The model under review builds one solid part; all positions refer to its coordinate system, in mm. Face numbers are marked on the shaded views. A direction names the side the tool comes from. Give positions to 0.01 mm unless a question says otherwise; leave off trailing zeros. Order: outer loops, then holes, each group sorted by start corner. A loop starts at its lowest first (then second) coordinate and runs counter-clockwise, first axis right, second up. Notation, with made-up numbers: (-38, -19.5) - (-33, -19.5) arc R19 ccw to (-33, -0.5) - close; hole circle Ø4 at (60.5, 80). An arc over 180 degrees is marked (long way). Use a Markdown table: item, result. Add a question column.
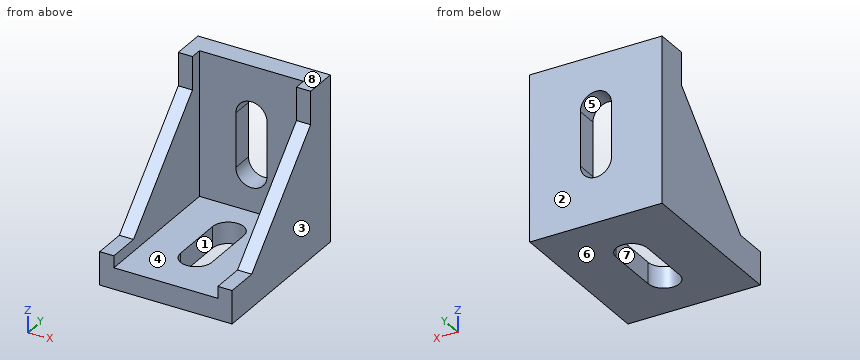
```python
from build123d import *

# Parameters (mm, degrees)
PAD_DEPTH            = 14
BOX_W                = 33
BOX_H                = 33
BOX_DEPTH            = 22
POCKET_DEPTH         = 4.5
POCKET001_DEPTH      = 4.5
BODY_ROLL_ANGLE      = 90
BODY_PLACEMENT_ANGLE = -90


with BuildPart() as part:
    # Sketch → Pad (new body, symmetric)
    with BuildSketch(Plane.XY):
        Polygon((0, 0), (0, 35), (7, 35), (7, 28), (28, 7), (35, 7), (35, 0), align=None)
    extrude(amount=PAD_DEPTH, both=True)

    # Box → Box (cut)
    with BuildSketch(Plane(origin=(4.5, 4.5, -11), x_dir=(1, 0, 0), z_dir=(0, 0, 1))):
        with Locations((16.5, 16.5)):
            Rectangle(BOX_W, BOX_H)
    extrude(amount=BOX_DEPTH, mode=Mode.SUBTRACT)

    # Sketch001 (on Face1 of Box) → Pocket (cut)
    with BuildSketch(Plane(origin=(0, 0, 0), x_dir=(0, -1, 0), z_dir=(-1, 0, 0))):
        with BuildLine():
            ThreePointArc((-24.2, 3.3), (-27.5, 0), (-24.2, -3.3))
            Line((-24.2, -3.3), (-12.8, -3.3))
            ThreePointArc((-12.8, -3.3), (-9.5, 0), (-12.8, 3.3))
            Line((-24.2, 3.3), (-12.8, 3.3))
        make_face()
    extrude(amount=-POCKET_DEPTH, mode=Mode.SUBTRACT)

    # Sketch002 (on Face2 of Pocket) → Pocket001 (cut)
    with BuildSketch(Plane.XZ):
        with BuildLine():
            ThreePointArc((12.8, 3.3), (9.5, 0), (12.8, -3.3))
            Line((12.8, -3.3), (24.2, -3.3))
            ThreePointArc((24.2, -3.3), (27.5, 0), (24.2, 3.3))
            Line((12.8, 3.3), (24.2, 3.3))
        make_face()
    extrude(amount=-POCKET001_DEPTH, mode=Mode.SUBTRACT)


with BuildPart() as part_1:
    # Body roll: moved
    add(part.part.rotate(Axis((0, 0, 0), (1, 0, 0)), BODY_ROLL_ANGLE))


with BuildPart() as part_2:
    # Body placement: moved
    add(part_1.part.rotate(Axis((0, 0, 0), (0, 0, 1)), BODY_PLACEMENT_ANGLE))


solid = part_2.part
```
Q1. We need section C-C (z = 16). Write out the cut boundary in (x, y), plus the area to 3 significant figures.
Q2. Wall thickness on probe 1 along X at (y, z) = (-2, 16.5); probe 2 along X at (y, z) = (-9, 11); probe 3 along Z at (x, y) = (0.5, -32): over which ranges is each line inside the solid? List them lowest first.
Q3. Clearance check with flat-ended pins moving along their axes: P1, Ø11, axis at x = 0.5, z = 22, coming from the -Y side; P2, Ø8, axis at x = -1.5, y = -12.5, coming from the +Z side; P3, Ø0.9, axis at x = -12.5, z = 33, coming from the -Y side. State where each tip first meets the part, or that it passes through.
Q4. Machinability: for the marked faces 4, 5, 6, 7 and 8, which of the approach directions +Z, -Z, +X, -X, +Y, -Y give a long, thin tool a straight path to every point of the face, cutting with its end or side? Answer none if there is none.
Q5. We need section A-A (x = 0). Write out the cut boundary in (y, z), plus the area to 3 significant figures.
Q6. We need section B-B (y = -3). Write out the cut boundary in (x, z).
Q7. Draft analysis for pull direction X (two halves, no side actions). For the marked faces 1, 2 and 3, state which applies: pulls with the +X half, pulls with the -X half, needs draft (parallel to the pull), parting line crosses it, or undercut.
Q8. We need section D-D (y = -22.5). Write out the cut boundary in (x, z), plus the area to 3 significant figures.
Here are the results:
| question | item | result |
|---|---|---|
| 1 | outline | (-14, -19) - (-11, -19) - (-11, -4.5) - (-3.3, -4.5) - (-3.3, 0) - (-14, 0) - close; (3.3, -4.5) - (11, -4.5) - (11, -19) - (14, -19) - (14, 0) - (3.3, 0) - close |
| 1 | area | 183 mm2 |
| 2 | probe 1 | -14 to -3.3, 3.3 to 14 |
| 2 | probe 2 | -14 to -11, 11 to 14 |
| 2 | probe 3 | 0 to 4.5 |
| 3 | P1 | y = -4.5 |
| 3 | P2 | z = 4.5 |
| 3 | P3 | y = -7 |
| 4 | face 4 | +Z, -Y |
| 4 | face 5 | +Y, -Y |
| 4 | face 6 | -Z, +X, -X, +Y, -Y |
| 4 | face 7 | +Z, -Z |
| 4 | face 8 | +Z, +X, -X, +Y, -Y |
| 5 | outline | (-35, 0) - (-27.5, 0) - (-27.5, 4.5) - (-35, 4.5) - close; (-9.5, 0) - (0, 0) - (0, 9.5) - (-4.5, 9.5) - (-4.5, 4.5) - (-9.5, 4.5) - close; (-4.5, 27.5) - (0, 27.5) - (0, 35) - (-4.5, 35) - close |
| 5 | area | 133 mm2 |
| 6 | outline | (-14, 0) - (14, 0) - (14, 35) - (-14, 35) - close; hole (-3.3, 12.8) arc R3.3 ccw to (3.3, 12.8) - (3.3, 24.2) arc R3.3 ccw to (-3.3, 24.2) - close |
| 7 | face 1 | undercut |
| 7 | face 2 | needs draft |
| 7 | face 3 | pulls with the +X half |
| 8 | outline | (-14, 0) - (-3.3, 0) - (-3.3, 4.5) - (-11, 4.5) - (-11, 12.5) - (-14, 12.5) - close; (3.3, 0) - (14, 0) - (14, 12.5) - (11, 12.5) - (11, 4.5) - (3.3, 4.5) - close |
| 8 | area | 144 mm2 |
